```python
from build123d import *

# Parameters (mm, degrees)
EXTRUDE_1_DEPTH = 3
SKETCH_2_W      = 30
SKETCH_2_H      = 30
EXTRUDE_2_DEPTH = 3


with BuildPart() as part:
    # 草图1 → 凸台-拉伸1 (new body)
    with BuildSketch(Plane(origin=(0, 0, 0), x_dir=(1, 0, 0), z_dir=(0, 1, 0))):
        Polygon((-21.213203436, 0), (0, -21.213203436), (21.213203436, 0), (0, 21.213203436), align=None)
    extrude(amount=EXTRUDE_1_DEPTH)

    # 草图2 → 凸台-拉伸2 (add)
    with BuildSketch(Plane(origin=(0, 0, 0), x_dir=(1, 0, 0), z_dir=(0, 1, 0))):
        Rectangle(SKETCH_2_W, SKETCH_2_H)
    extrude(amount=EXTRUDE_2_DEPTH)


solid = part.part
```
The listing builds one solid part. Answer for the finished solid, in the listing's coordinates (mm). A direction names the side the tool comes from. Round coordinates to 2 decimals unless told otherwise and drop trailing zeros. Loops run counter-clockwise (first coordinate to the right, second up) from the corner with the lowest first, then second, coordinate; pieces in that order, holes last.
1) A cutting plane is placed at A-A on y = 2.4. Determine the outline of the cut face in (x, z), plus the area to 3 significant figures.
Outcome:
outline: (-21.21, 0) - (-15, -6.21) - (-15, -15) - (-6.21, -15) - (0, -21.21) - (6.21, -15) - (15, -15) - (15, -6.21) - (21.21, 0) - (15, 6.21) - (15, 15) - (6.21, 15) - (0, 21.21) - (-6.21, 15) - (-15, 15) - (-15, 6.21) - close
area: 1,050 mm2
2) Given P1, Ø0.9, axis at y = 1, z = -12.5, coming from the -X side; P2, Ø1.5, axis at x = -9, y = 1, coming from the +Z side; P3, Ø1.5, axis at x = 10, y = 1.5, coming from the -Z side, each flat-ended and moving along its own axis, determine where each tip first touches the part or whether it passes through.
Outcome:
P1: stops at x = -15
P2: stops at z = 15
P3: stops at z = -15
3) Consider line 1 (X direction, y = 2.2, z = -6.5); line 2 (X direction, y = 0.7, z = -19). Determine where each line is inside the solid, lowest interval first.
Outcome:
line 1: x = -15 to 15
line 2: x = -2.21 to 2.21
4) For faces 1 (the face through (-11, 1, -15)), 2 (the face through (11, 1, 15)), 3 (the face through (-11, 1, 15)), 4 (the face through (0, 0, 0)), 5 (the face through (11, 1, -15)), determine the directions among +Z, -Z, +X, -X, +Y, -Y from which every point of the face is accessible in a straight line to the end or side of a thin tool.
Outcome:
face 1: -Z, -X, +Y, -Y
face 2: +Z, +X, +Y, -Y
face 3: +Z, -X, +Y, -Y
face 4: +Z, -Z, +X, -X, -Y
face 5: -Z, +X, +Y, -Y
5) A cutting plane is placed at B-B on x = 11.5. Determine the outline of the cut face in (y, z).
Outcome:
outline: (0, -15) - (3, -15) - (3, 15) - (0, 15) - close
6) A cutting plane is placed at C-C on z = -14.5. Determine the outline of the cut face in (x, y), plus the area to 3 significant figures.
Outcome:
outline: (-15, 0) - (15, 0) - (15, 3) - (-15, 3) - close
area: 90.0 mm2
